Verification items for the finished model (mm, model axes). A direction names the side the tool comes from. Round coordinates to 2 decimals unless told otherwise and drop trailing zeros. Loops run counter-clockwise (first coordinate to the right, second up) from the corner with the lowest first, then second, coordinate; pieces in that order, holes last. Notation, with made-up numbers: M 17.5,84.5 L 73.5,84.5 A29 cw 73.5,104.5 Z; hole C 68.25,-27 d8. An arc over 180 degrees is marked long. Answer as CSV lines item,"result".
```python
from build123d import *

# Parameters (mm, degrees)
PAD_DEPTH       = 20
SKETCH001_R     = 1.5
POCKET_DEPTH    = 22.501
FILLET_R        = 9
FILLET001_R     = 9
FILLET002_R     = 9
FILLET003_R     = 9
FILLET004_R     = 6
FILLET005_R     = 6
SKETCH002_R     = 1.5
POCKET001_DEPTH = 15.501
SKETCH003_R     = 1.25
POCKET002_DEPTH = 55.001155
SKETCH004_R     = 1
POCKET003_DEPTH = 54.95679


with BuildPart() as part:
    # Sketch → Pad (new body)
    with BuildSketch(Plane.XY):
        Polygon((-29.277703, 26.681208), (-17.777703, 26.681208), (-17.777703, 36.681208), (-13.777703, 36.681208), (-13.777703, 26.681208), (-2.277703, 26.681208), (-2.277703, -18.318792), (-6.777703, -18.318818), (-6.777703, -33.318818), (-12.777703, -33.318818), (-12.777703, -18.274582), (-18.777703, -18.274582), (-18.777703, -33.318792), (-24.777703, -33.318792), (-24.777703, -18.318792), (-29.277703, -18.318792), align=None)
    extrude(amount=PAD_DEPTH)

    # Sketch001 (on Face8 of Pad) → Pocket (cut, through all)
    with BuildSketch(Plane.YZ.offset(-6.777703)):
        with Locations((-27.212769, 10.156303)):
            Circle(SKETCH001_R)
    extrude(amount=-POCKET_DEPTH, mode=Mode.SUBTRACT)

    # Fillet
    fillet_edges = [part.edges().sort_by_distance(p)[0] for p in [
        (-21.777703, -33.318792, 20),
    ]]
    fillet(fillet_edges, radius=FILLET_R)

    # Fillet001
    fillet001_edges = [part.edges().sort_by_distance(p)[0] for p in [
        (-21.777703, -33.318792, 0),
    ]]
    fillet(fillet001_edges, radius=FILLET001_R)

    # Fillet002
    fillet002_edges = [part.edges().sort_by_distance(p)[0] for p in [
        (-9.777703, -33.318818, 20),
    ]]
    fillet(fillet002_edges, radius=FILLET002_R)

    # Fillet003
    fillet003_edges = [part.edges().sort_by_distance(p)[0] for p in [
        (-9.777703, -33.318818, 0),
    ]]
    fillet(fillet003_edges, radius=FILLET003_R)

    # Fillet004
    fillet004_edges = [part.edges().sort_by_distance(p)[0] for p in [
        (-15.777703, 36.681208, 20),
    ]]
    fillet(fillet004_edges, radius=FILLET004_R)

    # Fillet005
    fillet005_edges = [part.edges().sort_by_distance(p)[0] for p in [
        (-15.777703, 36.681208, 0),
    ]]
    fillet(fillet005_edges, radius=FILLET005_R)

    # Sketch002 (on Face8 of Fillet005) → Pocket001 (cut, through all)
    with BuildSketch(Plane(origin=(-17.777703, 0, 0), x_dir=(0, -1, 0), z_dir=(-1, 0, 0))):
        with Locations((-31.403757, 9.939318)):
            Circle(SKETCH002_R)
    extrude(amount=-POCKET001_DEPTH, mode=Mode.SUBTRACT)

    # Sketch003 (on Face12 of Pocket001) → Pocket002 (cut, through all)
    with BuildSketch(Plane(origin=(0.000105, -18.318779, 0), x_dir=(1, 6e-06, 0), z_dir=(6e-06, -1, 0))):
        with Locations((-27.20172, 5.947487)):
            Circle(SKETCH003_R)
        with Locations((-4.360133, 6.030852)):
            Circle(SKETCH003_R)
    extrude(amount=-POCKET002_DEPTH, mode=Mode.SUBTRACT)

    # Sketch004 (on Face20 of Pocket002) → Pocket003 (cut, through all)
    with BuildSketch(Plane.XZ.offset(18.274582)):
        with Locations((-15.464924, 16.684162)):
            Circle(SKETCH004_R)
    extrude(amount=-POCKET003_DEPTH, mode=Mode.SUBTRACT)


solid = part.part
```
1) Section check B-B (y = -26.5). Record the cut outline in (x, z), plus the area to 3 significant figures.
Here are the results:
outline,"M -24.78,0.27 L -18.78,0.27 L -18.78,8.84 L -24.78,8.84 Z; M -24.78,11.48 L -18.78,11.48 L -18.78,19.73 L -24.78,19.73 Z; M -12.78,0.27 L -6.78,0.27 L -6.78,8.84 L -12.78,8.84 Z; M -12.78,11.48 L -6.78,11.48 L -6.78,19.73 L -12.78,19.73 Z"
area,"202 mm^2"
2) Set-up check for faces 4 (the flat face through (-16, -18.275, 10)), 5 (the flat face through (-27, -18.319, 10)), 6 (the flat face through (-6.778, -24, 10)), 7 (the flat face through (-24, 26.681, 10)): record each of +Z, -Z, +X, -X, +Y, -Y from which the full face is reachable in a straight line by a thin tool's end or side.
Here are the results:
face 4,"+Z, -Z, -Y"
face 5,"+Z, -Z, -X, -Y"
face 6,"+Z, -Z, +X, -Y"
face 7,"+Z, -Z, -X, +Y"
3) Section check C-C (x = -21). Record the cut outline in (y, z), plus the area to 3 significant figures.
Here are the results:
outline,"M -33.32,9 A9 ccw -24.32,0 L 26.68,0 L 26.68,20 L -24.32,20 A9 ccw -33.32,11 Z; hole C -27.21,10.16 d3"
area,"1,160 mm^2"
4) Section check A-A (x = -15.75). Record the cut outline in (y, z).
Here are the results:
outline,"M -18.27,0 L 30.68,0 A6 ccw 36.68,6 L 36.68,14 A6 ccw 36.43,15.73 L -18.27,15.73 Z; M -18.27,17.64 L 35.45,17.64 A6 ccw 30.68,20 L -18.27,20 Z; hole C 31.4,9.94 d3"
5) Section check D-D (z = 1). Record the cut outline in (x, y), plus the area to 3 significant figures.
Here are the results:
outline,"M -29.28,-18.32 L -24.78,-18.32 L -24.78,-28.44 L -18.78,-28.44 L -18.78,-18.27 L -12.78,-18.27 L -12.78,-28.44 L -6.78,-28.44 L -6.78,-18.32 L -2.28,-18.32 L -2.28,26.68 L -13.78,26.68 L -13.78,34 L -17.78,34 L -17.78,26.68 L -29.28,26.68 Z"
area,"1,370 mm^2"
6) Go/stop test with flat-tipped pins: pin 1 (3 mm diameter, centred on x = -16, y = -6, fed in from -Z); pin 2 (11 mm diameter, centred on y = 34, z = 6, fed in from -X); pin 3 (2 mm diameter, centred on x = -4.36, z = 6.03, fed in from +Y); pin 4 (3.5 mm diameter, centred on x = -9, z = 12.5, fed in from +Y). Record where each tip stops, or that it passes through.
Here are the results:
pin 1,"stops at z = 0"
pin 2,"stops at x = -17.78"
pin 3,"passes through"
pin 4,"stops at y = 26.68"
7) Draft check along X on faces 1 (the flat face through (-12.778, -24, 10)), 2 (the cylindrical face through (-15.806, 32.594, 9.027)), 3 (the flat face through (-29.278, 4, 10)). Enter one of: +X half, -X half, draft (parallel to the pull), parting line (faces both ways), or undercut.
Here are the results:
face 1,"undercut"
face 2,"draft"
face 3,"-X half"
8) Material ranges on probe 1 along Z at (x, y) = (-27, 0.5); probe 2 along X at (y, z) = (-29.5, 9.75); probe 3 along Y at (x, z) = (-15.5, 12.25), recorded low to high.
Here are the results:
probe 1,"z = 0 to 4.71, 7.18 to 20"
probe 2,"x = -24.78 to -18.78, -12.78 to -6.78"
probe 3,"y = -18.27 to 36.68"
